Geometry: final body of the model. Coordinates: model frame, mm. A direction names the side the tool comes from. Coordinates: 2 decimals unless noted, no trailing zeros. Loops run counter-clockwise (first coordinate to the right, second up) from the corner with the lowest first, then second, coordinate; pieces in that order, holes last. Notation, with made-up numbers: (55, 58) - (98, 58) arc R20 ccw to (98, 89) - close; hole circle Ø11 at (-3, 41). An arc over 180 degrees is marked (long way). Answer in a Markdown table with one row per item.
from build123d import *

# Parameters (mm, degrees)
SKETCH1_R           = 45
BOSS_EXTRUDE1_DEPTH = 34
SKETCH2_R           = 45
BOSS_EXTRUDE2_DEPTH = 6
BOSS_EXTRUDE3_DEPTH = 34
FILLET1_R           = 6
CHAMFER1_SIZE       = 6
FILLET2_R           = 3
FILLET3_R           = 6.35
SKETCH4_R           = 3.175
CUT_EXTRUDE1_DEPTH  = 34


with BuildPart() as part:
    # Sketch1 → Boss-Extrude1 (new body)
    with BuildSketch(Plane(origin=(0, 0, 0), x_dir=(1, 0, 0), z_dir=(0, 1, 0))):
        Circle(SKETCH1_R)
        Polygon((37.816442632, 0), (18.908221316, 32.75), (-18.908221316, 32.75), (-37.816442632, 0), (-18.908221316, -32.75), (18.908221316, -32.75), align=None, mode=Mode.SUBTRACT)
    extrude(amount=BOSS_EXTRUDE1_DEPTH)

    # Sketch2 → Boss-Extrude2 (add)
    with BuildSketch(Plane(origin=(0, 34, 0), x_dir=(1, 0, 0), z_dir=(0, 1, 0))):
        Circle(SKETCH2_R)
    extrude(amount=BOSS_EXTRUDE2_DEPTH)

    # Sketch3 → Boss-Extrude3 (add)
    with BuildSketch(Plane(origin=(0, 40, 0), x_dir=(1, 0, 0), z_dir=(0, 1, 0))):
        Polygon((28.867513459, 0), (14.43375673, 25), (-14.43375673, 25), (-28.867513459, 0), (-14.43375673, -25), (14.43375673, -25), align=None)
    extrude(amount=BOSS_EXTRUDE3_DEPTH)

    # Fillet1
    fillet1_edges = [part.edges().sort_by_distance(p)[0] for p in [
        (21.650635095, 40, 12.5),
        (21.650635095, 40, -12.5),
        (0, 40, -25),
        (-21.650635095, 40, -12.5),
        (-21.650635095, 40, 12.5),
        (0, 40, 25),
    ]]
    fillet(fillet1_edges, radius=FILLET1_R)

    # Chamfer1
    chamfer1_edges = [part.edges().sort_by_distance(p)[0] for p in [
        (-45, 40, 0),
    ]]
    chamfer(chamfer1_edges, length=CHAMFER1_SIZE)

    # Fillet2
    fillet2_edges = [part.edges().sort_by_distance(p)[0] for p in [
        (-45, 0, 0),
    ]]
    fillet(fillet2_edges, radius=FILLET2_R)

    # Fillet3
    fillet3_edges = [part.edges().sort_by_distance(p)[0] for p in [
        (37.816442632, 17, 0),
        (18.908221316, 17, -32.75),
        (-18.908221316, 17, -32.75),
        (-37.816442632, 17, 0),
        (-18.908221316, 17, 32.75),
        (18.908221316, 17, 32.75),
    ]]
    fillet(fillet3_edges, radius=FILLET3_R)

    # Sketch4 → Cut-Extrude1 (cut)
    with BuildSketch(Plane.XZ):
        with Locations((17.320721316, 30.000369343)):
            Circle(SKETCH4_R)
        with Locations((34.641442632, 0)):
            Circle(SKETCH4_R)
        with Locations((17.320721316, -30.000369343)):
            Circle(SKETCH4_R)
        with Locations((-17.320721316, -30.000369343)):
            Circle(SKETCH4_R)
        with Locations((-34.641442632, 0)):
            Circle(SKETCH4_R)
        with Locations((-17.320721316, 30.000369343)):
            Circle(SKETCH4_R)
    extrude(amount=-CUT_EXTRUDE1_DEPTH, mode=Mode.SUBTRACT)


solid = part.part
(1) Pull-direction query (Z, two-part tool) for faces 5 (the face through (-37.816, 16.762, 0.047)), 6 (the face through (0, 74, 0)), 7 (the face through (21.75, 59.8, -12.33)), 8 (the face through (18.87, 16.76, -32.77)); classes: pulls with the +Z half, pulls with the -Z half, needs draft (parallel to the pull), parting line crosses it, or undercut.
Verdict:
| item | result |
|---|---|
| face 5 | undercut |
| face 6 | needs draft |
| face 7 | pulls with the -Z half |
| face 8 | undercut |
(2) First-contact query: pin 1 Ø22.5 at (x, y) = (-6, 58) entering from +Z; pin 2 Ø1.5 at (x, y) = (21, 8) entering from -Z; pin 3 Ø1.5 at (x, y) = (24, 58) entering from -Z. Flat tips, straight axial feed; report the tip coordinate or a pass-through.
Verdict:
| item | result |
|---|---|
| pin 1 | stops at z = 25 |
| pin 2 | stops at z = -40.19 |
| pin 3 | stops at z = -9.73 |
(3) Access query for faces 1 (the face through (0, 60, -25)), 2 (the face through (-28, 0, -19)), 3 (the face through (-18.949, 16.762, -32.726)), 4 (the face through (-21.75, 59.8, 12.33)). Directions: +Z, -Z, +X, -X, +Y, -Y. A direction counts if a zero-diameter tool reaches every point of the face in a straight line with its end or side. Return the directions, or none.
Verdict:
| item | result |
|---|---|
| face 1 | -Z, +X, -X, +Y |
| face 2 | +Z, -Z, +X, -X, -Y |
| face 3 | -Y |
| face 4 | +Z, -X, +Y |
(4) Cut plane B-B on y = 58. Output: boundary loops of the cut face in (x, z).
Verdict:
| item | result |
|---|---|
| outline | (-28.87, 0) - (-14.43, -25) - (14.43, -25) - (28.87, 0) - (14.43, 25) - (-14.43, 25) - close |
(5) Ray query, probe 1 along Y at (x, z) = (-6.5, -7); probe 2 along Z at (x, y) = (7, 13); probe 3 along Y at (x, z) = (-31, -22). Return the intervals inside material, ascending.
Verdict:
| item | result |
|---|---|
| probe 1 | y = 34 to 74 |
| probe 2 | z = -44.45 to -32.75, 32.75 to 44.45 |
| probe 3 | y = 0 to 40 |
(6) Cut plane A-A on x = 0. Output: boundary loops of the cut face in (y, z).
Verdict:
| item | result |
|---|---|
| outline | (0, -42) arc R3 ccw to (3, -45) - (34, -45) - (40, -39) - (40, -31) arc R6 cw to (46, -25) - (74, -25) - (74, 25) - (46, 25) arc R6 cw to (40, 31) - (40, 39) - (34, 45) - (3, 45) arc R3 ccw to (0, 42) - (0, 32.75) - (34, 32.75) - (34, -32.75) - (0, -32.75) - close |
